Could you check a few things on this model? Use its own coordinates, in mm. Face numbers are marked on the shaded views. A direction names the side the tool comes from. Round coordinates to 2 decimals unless told otherwise and drop trailing zeros. Order: outer loops, then holes, each group sorted by start corner. A loop starts at its lowest first (then second) coordinate and runs counter-clockwise, first axis right, second up.
```python
from build123d import *

# Parameters (mm, degrees)
SKIZZE1_R                        = 22.5
SEITE1_DEPTH                     = 2
SKIZZE2_R                        = 20.5
LAUFFL_CHE_DEPTH                 = 8
SKIZZE5_R                        = 22.5
SEITE_2_DEPTH                    = 2
BOHRUNG_DEPTH                    = 100
BOHRUNG_DEPTH_BACK               = 34.35416016
SKIZZE7_R                        = 2.5
SKIZZE9_R                        = 10
ZAPFEN_DEPTH                     = 25
SKIZZE10_R                       = 19
SEITENTEIL3_DEPTH                = 2
SKIZZE12_R                       = 17.5
ZAHNFL_CHE_DEPTH                 = 8
SKIZZE13_R                       = 19
SEITENTEIL4_DEPTH                = 2
F_12_0_12_DURCHMESSER_BOHRUNG1_D = 12


with BuildPart() as part:
    # Skizze1 → Seite1 (new body)
    with BuildSketch(Plane.XY):
        Circle(SKIZZE1_R)
    extrude(amount=SEITE1_DEPTH)

    # Skizze2 → Lauffläche (add)
    with BuildSketch(Plane.XY):
        Circle(SKIZZE2_R)
    extrude(amount=LAUFFL_CHE_DEPTH)

    # Skizze5 → Seite 2 (add)
    with BuildSketch(Plane.XY.offset(8)):
        Circle(SKIZZE5_R)
    extrude(amount=SEITE_2_DEPTH)

    # Skizze7 → Bohrung (cut, two sides: drawn at the far end of the back side and taken through both)
    with BuildSketch(Plane.XY.offset(-BOHRUNG_DEPTH_BACK)):
        Circle(SKIZZE7_R)
    extrude(amount=BOHRUNG_DEPTH + BOHRUNG_DEPTH_BACK, mode=Mode.SUBTRACT)

    # Skizze9 → Zapfen (add)
    with BuildSketch(Plane.XY.offset(10)):
        Circle(SKIZZE9_R)
    extrude(amount=ZAPFEN_DEPTH)

    # Skizze10 → Seitenteil3 (add)
    with BuildSketch(Plane.XY.offset(35)):
        Circle(SKIZZE10_R)
    extrude(amount=SEITENTEIL3_DEPTH)

    # Skizze12 → Zahnfläche (add)
    with BuildSketch(Plane.XY.offset(37)):
        Circle(SKIZZE12_R)
    extrude(amount=ZAHNFL_CHE_DEPTH)

    # Skizze13 → Seitenteil4 (add)
    with BuildSketch(Plane.XY.offset(45)):
        Circle(SKIZZE13_R)
    extrude(amount=SEITENTEIL4_DEPTH)

    # Ø12.0 (12) Durchmesser Bohrung1 (through all)
    with Locations(Plane(origin=(0, 0, 0), x_dir=(-1, 0, 0), z_dir=(0, 0, -1))):
        with Locations((0, 0)):
            Hole(F_12_0_12_DURCHMESSER_BOHRUNG1_D / 2)


solid = part.part
```
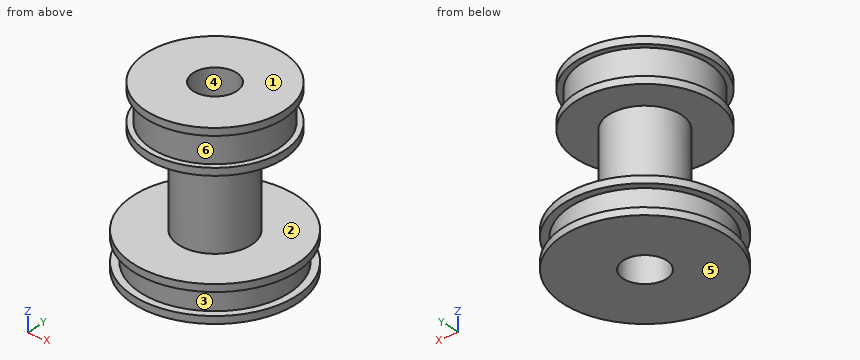
Q1. Imagine slicing it at D-D, the plane x = 7. Please give me the cut outline in (y, z), then the cut area to 3 significant figures.
Q2. We'd pull the mould along Z, two halves only. Please class the marked faces 3, 4, 5 and 6: released by +Z, released by -Z, zero draft, split by the parting line, or undercut.
Q3. For P1, Ø19, axis at x = 4, y = 0.5, coming from the -Z side; P2, Ø2, axis at y = 16.5, z = 5, coming from the +X side; P3, Ø1, axis at y = 17, z = 36, coming from the -X side; P4, Ø10, axis at x = -9, z = 32.5, coming from the +Y side, each with a flat end and sliding along its axis, tell me the tip position at first contact or that it passes through.
Q4. Imagine slicing it at C-C, the plane z = 43.5. Please give me the cut outline in (x, y).
Q5. For the marked faces 1 and 2, which set-ups out of +Z, -Z, +X, -X, +Y, -Y let a thin tool reach every point of the face, with its end or its side?
Q6. I need wall thicknesses on L1, parallel to Z at x = 17, y = -6.5; L2, parallel to Y at x = 0, z = 24; L3, parallel to Z at x = -12.5, y = 2.5. Which ranges of each line are inside material? Lowest first, please.
Filled in:
1. outline: (-21.38, 0) - (21.38, 0) - (21.38, 2) - (19.27, 2) - (19.27, 8) - (21.38, 8) - (21.38, 10) - (7.14, 10) - (7.14, 35) - (17.66, 35) - (17.66, 37) - (16.04, 37) - (16.04, 45) - (17.66, 45) - (17.66, 47) - (-17.66, 47) - (-17.66, 45) - (-16.04, 45) - (-16.04, 37) - (-17.66, 37) - (-17.66, 35) - (-7.14, 35) - (-7.14, 10) - (-21.38, 10) - (-21.38, 8) - (-19.27, 8) - (-19.27, 2) - (-21.38, 2) - close
1. area: 1,160 mm2
2. face 3: undercut
2. face 4: zero draft
2. face 5: released by -Z
2. face 6: undercut
3. P1: stops at z = 0
3. P2: stops at x = 13.42
3. P3: stops at x = -9.42
3. P4: stops at y = 18.42
4. outline: circle Ø35 at (0, 0); hole circle Ø12 at (0, 0)
5. face 1: +Z, +X, -X, +Y, -Y
5. face 2: none
6. L1: z = 0 to 10, 35 to 37, 45 to 47
6. L2: y = -10 to -6, 6 to 10
6. L3: z = 0 to 10, 35 to 47
